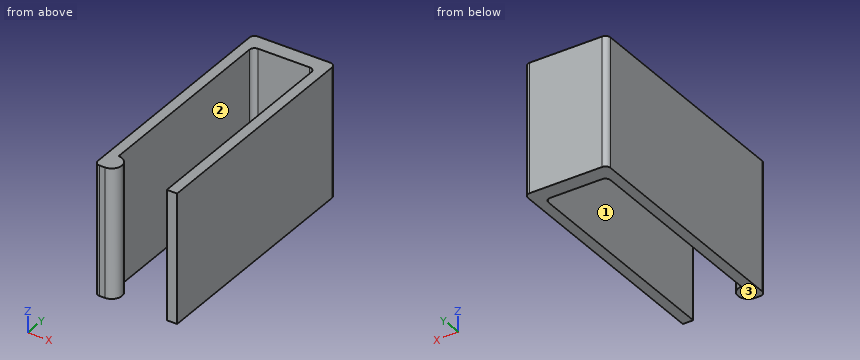
from build123d import *

# Parameters (mm, degrees)
PAD_DEPTH = 25
FILLET_R  = 1


with BuildPart() as part:
    # Sketch → Pad (new body)
    with BuildSketch(Plane.XY):
        with BuildLine():
            Line((8, 0), (8, -45))
            Line((8, -45), (6, -45))
            Line((6, -45), (6, -3))
            ThreePointArc((6, -3), (5.707107, -2.292893), (5, -2))
            Line((-5, -2), (5, -2))
            ThreePointArc((-5, -2), (-5.707107, -2.292893), (-6, -3))
            Line((-6, -3), (-6, -41))
            ThreePointArc((-6, -45), (-4, -43), (-6, -41))
            Line((-6, -45), (-8, -45))
            Line((-8, -45), (-8, 0))
            ThreePointArc((-7, 1), (-7.707107, 0.707107), (-8, 0))
            Line((-7, 1), (7, 1))
            ThreePointArc((8, 0), (7.707107, 0.707107), (7, 1))
        make_face()
    extrude(amount=PAD_DEPTH)

    # Fillet
    fillet_edges = [part.edges().sort_by_distance(p)[0] for p in [
        (-8, -45, 12.5),
    ]]
    fillet(fillet_edges, radius=FILLET_R)


solid = part.part
For this review, take the finished solid that the model builds, in its own axes (mm). Face numbers are marked on the shaded views. A direction names the side the tool comes from. Round coordinates to 2 decimals unless told otherwise and drop trailing zeros. Order: outer loops, then holes, each group sorted by start corner. A loop starts at its lowest first (then second) coordinate and runs counter-clockwise, first axis right, second up. Notation, with made-up numbers: M 48.25,-13 L 62.25,-13 A32 cw 62.25,26 Z; hole C -27,70.25 d4. An arc over 180 degrees is marked long. Use a Markdown table: item, result. Add a question column.
Item 1: To check wall thickness, follow line 1 along X through (y, z) = (-3, 10); line 2 along Y through (x, z) = (-3.5, 20); line 3 along X through (y, z) = (-2.5, 2.5). State the ranges of each line that lie inside material, in increasing order.
Item 2: Add section A-A, the plane y = -10. Give the boundary of the cut face in (x, z), then the cut area to 3 significant figures.
Item 3: Add section D-D, the plane x = 0.5. Give the boundary of the cut face in (y, z), then the cut area to 3 significant figures.
Item 4: Add section B-B, the plane x = -4.5. Give the boundary of the cut face in (y, z).
Item 5: Insertion check: pin 1 (6 mm diameter, centred on x = -5, y = -29, fed in from +Z). The pin has a flat end and moves straight along its axis. Give the tip position at first contact, or say it passes through.
Item 6: Tool access review of the marked faces 1, 2 and 3: name each direction out of +Z, -Z, +X, -X, +Y, -Y from which nothing blocks a thin tool from reaching the whole face with its end or side.
Item 7: Add section C-C, the plane z = 8. Give the boundary of the cut face in (x, y).
Geometry results:
| question | item | result |
|---|---|---|
| 1 | line 1 | x = -8 to -6, 6 to 8 |
| 1 | line 2 | y = -2 to 1 |
| 1 | line 3 | x = -8 to -5.87, 5.87 to 8 |
| 2 | outline | M -8,0 L -6,0 L -6,25 L -8,25 Z; M 6,0 L 8,0 L 8,25 L 6,25 Z |
| 2 | area | 100 mm² |
| 3 | outline | M -2,0 L 1,0 L 1,25 L -2,25 Z |
| 3 | area | 75.0 mm² |
| 4 | outline | M -44.32,0 L -41.68,0 L -41.68,25 L -44.32,25 Z; M -2,0 L 1,0 L 1,25 L -2,25 Z |
| 5 | pin 1 | stops at z = 25 |
| 6 | face 1 | +Z, -Z, -Y |
| 6 | face 2 | +Z, -Z |
| 6 | face 3 | -Z, +X, -X, +Y, -Y |
| 7 | outline | M -8,-44 A1 ccw -7,-45 L -6,-45 A2 ccw -6,-41 L -6,-3 A1 cw -5,-2 L 5,-2 A1 cw 6,-3 L 6,-45 L 8,-45 L 8,0 A1 ccw 7,1 L -7,1 A1 ccw -8,0 Z |
